```python
from build123d import *

# Parameters (mm, degrees)
F1_DEPTH = 100
F3_DEPTH = 10
F5_DEPTH = 12
F6_SIZE  = 1.19999


# Not quite as in the source:
# - a fillet or chamfer is up to 0.001 mm smaller than in the source, because OpenCascade refuses the exact size


with BuildPart() as f1:
    # F0 (on Top) → F1 (new body)
    with BuildSketch(Plane.XY):
        with BuildLine():
            Line((-12.0897765349, -15.731314094), (27.9102234651, -15.731314094))
            ThreePointArc((27.9102234651, -15.731314094), (35.186552736, 4.9027765722), (25.0045970812, 24.268685906))
            Line((25.0045970812, 24.268685906), (5.1992357064, 21.4852238868))
            ThreePointArc((5.1992357064, 21.4852238868), (0.7654520553, 17.832613514), (-4.5033702016, 20.1216115537))
            Line((-4.5033702016, 20.1216115537), (-14.406050889, 18.7298805441))
            ThreePointArc((-14.406050889, 18.7298805441), (-19.3764079278, 1.0873626828), (-12.0897765349, -15.731314094))
        make_face()
        with BuildLine():
            ThreePointArc((-11.0175789214, -13.331314094), (-16.9820661814, 1.2521155975), (-13.0181733872, 16.5013478326))
            Line((-13.0181733872, 16.5013478326), (-5.4545185869, 17.5643501916))
            ThreePointArc((-5.4545185869, 17.5643501916), (1.0994674976, 15.455970149), (6.8184149763, 19.2891985189))
            Line((6.8184149763, 19.2891985189), (24.284750464, 21.7439318875))
            ThreePointArc((24.284750464, 21.7439318875), (32.7925833849, 4.7326981573), (26.8380258517, -13.331314094))
            Line((26.8380258517, -13.331314094), (-11.0175789214, -13.331314094))
        make_face(mode=Mode.SUBTRACT)
    extrude(amount=F1_DEPTH)

    # F2 (on face) → F3 (cut)
    with BuildSketch(Plane(origin=(0, 0, 0), x_dir=(1, 0, 0), z_dir=(0, 0, -1))):
        with BuildLine():
            Line((27.9102234651, 15.731314094), (-12.0897765349, 15.731314094))
            ThreePointArc((-12.0897765349, 15.731314094), (-19.3764079278, -1.0873626828), (-14.406050889, -18.7298805441))
            Line((-14.406050889, -18.7298805441), (-4.5033702016, -20.1216115537))
            ThreePointArc((-4.5033702016, -20.1216115537), (0.7654520553, -17.832613514), (5.1992357064, -21.4852238868))
            Line((5.1992357064, -21.4852238868), (25.0045970812, -24.268685906))
            ThreePointArc((25.0045970812, -24.268685906), (35.186552736, -4.9027765722), (27.9102234651, 15.731314094))
        make_face()
        with BuildLine():
            ThreePointArc((6.0462768814, -20.3924746735), (0.9324597764, -16.6442918315), (-5.0163959343, -18.837717402))
            Line((-5.0163959343, -18.837717402), (-13.7193495518, -17.6145970362))
            ThreePointArc((-13.7193495518, -17.6145970362), (-18.1792377522, -1.1697483945), (-11.5610592762, 14.531314094))
            Line((-11.5610592762, 14.531314094), (27.3815062065, 14.531314094))
            ThreePointArc((27.3815062065, 14.531314094), (33.9895674633, -4.8177466261), (24.6519111864, -23.0073260489))
            Line((24.6519111864, -23.0073260489), (6.0462768814, -20.3924746735))
        make_face(mode=Mode.SUBTRACT)
    extrude(amount=-F3_DEPTH, mode=Mode.SUBTRACT)

    # F4 (on face) → F5 (cut)
    with BuildSketch(Plane.XY.offset(100)):
        with BuildLine():
            Line((-5.0163959343, 18.837717402), (-13.7193495518, 17.6145970362))
            ThreePointArc((-13.7193495518, 17.6145970362), (-18.1792377522, 1.1697483945), (-11.5610592762, -14.531314094))
            Line((-11.5610592762, -14.531314094), (27.3815062065, -14.531314094))
            ThreePointArc((27.3815062065, -14.531314094), (33.9895674633, 4.8177466261), (24.6519111864, 23.0073260489))
            Line((24.6519111864, 23.0073260489), (6.0462768814, 20.3924746735))
            ThreePointArc((6.0462768814, 20.3924746735), (0.9324597764, 16.6442918315), (-5.0163959343, 18.837717402))
        make_face()
        with BuildLine():
            ThreePointArc((24.284750464, 21.7439318875), (32.7925833849, 4.7326981573), (26.8380258517, -13.331314094))
            Line((26.8380258517, -13.331314094), (-11.0175789214, -13.331314094))
            ThreePointArc((-11.0175789214, -13.331314094), (-16.9820661814, 1.2521155975), (-13.0181733872, 16.5013478326))
            Line((-13.0181733872, 16.5013478326), (-5.4545185869, 17.5643501916))
            ThreePointArc((-5.4545185869, 17.5643501916), (1.0994674976, 15.455970149), (6.8184149763, 19.2891985189))
            Line((6.8184149763, 19.2891985189), (24.284750464, 21.7439318875))
        make_face(mode=Mode.SUBTRACT)
    extrude(amount=-F5_DEPTH, mode=Mode.SUBTRACT)

    # F6 (size 1.2 in the source; OpenCascade refuses exactly that, so slightly less here)
    f6_edges = [f1.edges().sort_by_distance(p)[0] for p in [
        (15.349094, 21.6999, 10),
        (33.989567, 4.817747, 10),
        (0.93246, 16.644292, 10),
        (-9.367873, 18.226157, 10),
        (-18.179238, 1.169748, 10),
        (7.910223, -14.531314, 10),
        (-18.179238, 1.169748, 88),
        (-9.367873, 18.226157, 88),
        (0.93246, 16.644292, 88),
        (15.349094, 21.6999, 88),
        (7.910223, -14.531314, 88),
        (33.989567, 4.817747, 88),
    ]]
    chamfer(f6_edges, length=F6_SIZE)


solid = f1.part
```
Source: CAD feature listing. Evaluate the final solid. Frame: model axes, mm. A direction names the side the tool comes from. Give positions to 0.01 mm unless a question says otherwise; leave off trailing zeros. Order: outer loops, then holes, each group sorted by start corner. A loop starts at its lowest first (then second) coordinate and runs counter-clockwise, first axis right, second up.
(1) Section query A-A (z = 50.5). Return the cut outline in (x, y).
(2) Access query for faces 1 (the face through (34.01, 4.52, 4.34)), 2 (the face through (4, 17, 0)), 3 (the face through (8, -15.731, 54)), 4 (the face through (8, -14.531, 95)), 5 (the face through (8, -13.331, 43)). Directions: +Z, -Z, +X, -X, +Y, -Y. A direction counts if a zero-diameter tool reaches every point of the face in a straight line with its end or side. Return the directions, or none.
(3) Material intervals for line 1 along Y through (x, z) = (0, 47.5); line 2 along X through (y, z) = (18.5, 25); line 3 along Y through (x, z) = (2, 78), sorted ascending.
(4) Contact query for flat-ended pins moving along their axis: P1, Ø10, axis at y = 12, z = 33.5, coming from the +X side; P2, Ø5, axis at y = 14.5, z = 21, coming from the +X side; P3, Ø12, axis at x = 11.5, z = 95.5, coming from the +Y side. Output: stop coordinate, or through.
(5) Pull-direction query (X, two-part tool) for faces 6 (the face through (1.001, 15.443, 43.384)), 7 (the face through (-18.194, 1.412, 4.338)), 8 (the face through (8, -15, 100)); classes: +X half, -X half, draft (parallel to the pull), parting line (faces both ways), or undercut.
Outcome:
1. outline: (-14.41, 18.73) arc R27.35 ccw to (-12.09, -15.73) - (27.91, -15.73) arc R27.35 ccw to (25, 24.27) - (5.2, 21.49) arc R5.5 cw to (-4.5, 20.12) - close; hole (-13.02, 16.5) arc R24.95 ccw to (-11.02, -13.33) - (26.84, -13.33) arc R24.95 ccw to (24.28, 21.74) - (6.82, 19.29) arc R7.9 cw to (-5.45, 17.56) - close
2. face 1: -Z, +X
2. face 2: -Z, +X, -X, +Y, -Y
2. face 3: +Z, -Z, +X, -X, -Y
2. face 4: +Z
2. face 5: +Z, -Z
3. line 1: y = -15.73 to -13.33, 15.38 to 17.78
3. line 2: x = -14.57 to -2.72, 2.72 to 6.29, 27.4 to 30.39
3. line 3: y = -15.73 to -13.33, 15.64 to 18.16
4. P1: stops at x = 34.95
4. P2: stops at x = 33.71
4. P3: stops at y = 23.21
5. face 6: undercut
5. face 7: -X half
5. face 8: draft
